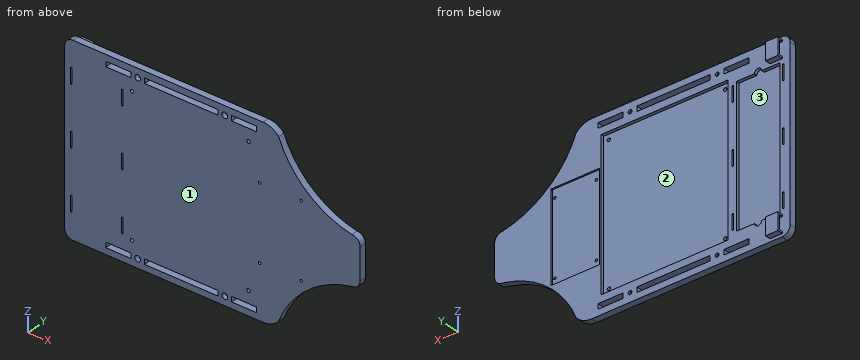
```python
from build123d import *

# Parameters (mm, degrees)
SALIENTE_EXTRUIR1_DEPTH = 6.35
CROQUIS2_R              = 1.825
CROQUIS2_W              = 63.849825594
CROQUIS2_H              = 5
CROQUIS2_W_2            = 24.299825594
CORTAR_EXTRUIR1_DEPTH   = 220.409920137
CORTAR_EXTRUIR2_DEPTH   = 3.175
CROQUIS4_W              = 45
CROQUIS4_H              = 80.85
CORTAR_EXTRUIR3_DEPTH   = 1.5
CROQUIS5_R              = 1.25
CORTAR_EXTRUIR4_DEPTH   = 220.371632292
CROQUIS7_W              = 44.995929737
CROQUIS7_H              = 3.9
CORTAR_EXTRUIR5_DEPTH   = 1.5
CROQUIS8_W              = 1.5
CROQUIS8_H              = 15
CORTAR_EXTRUIR6_DEPTH   = 220.409920137
CROQUIS9_W              = 123
CROQUIS9_H              = 144
CORTAR_EXTRUIR7_DEPTH   = 3.175
CROQUIS10_R             = 2.8
CORTAR_EXTRUIR8_DEPTH   = 4.35
CROQUIS11_R             = 1.65
CORTAR_EXTRUIR9_DEPTH   = 220.34099293
CROQUIS13_W             = 12.1
CROQUIS13_H             = 17
SALIENTE_EXTRUIR2_DEPTH = 5.5
CROQUIS14_W             = 13.5
CROQUIS14_H             = 3.5
CORTAR_EXTRUIR10_DEPTH  = 12.1
CROQUIS15_W             = 13.5
CROQUIS15_H             = 3.5
CORTAR_EXTRUIR11_DEPTH  = 12.1
CORTAR_EXTRUIR12_DEPTH  = 220.409920137
CORTAR_EXTRUIR15_DEPTH  = 1.5
CROQUIS19_W             = 7.395174406
CROQUIS19_H             = 5
CORTAR_EXTRUIR16_DEPTH  = 220.409920137


with BuildPart() as part:
    # Croquis1 → Saliente-Extruir1 (new body)
    with BuildSketch(Plane(origin=(0, 0, 0), x_dir=(1, 0, 0), z_dir=(0, 1, 0))):
        with BuildLine():
            Line((0, 0), (200, 0))
            Line((200, 0), (200, 15.2))
            ThreePointArc((200, 15.2), (197.701163079, 20.938172036), (191.9990235, 23.3249845))
            ThreePointArc((191.9990235, 23.3249845), (148.666739026, 44.032184001), (120.7781513, 83.1307986))
            ThreePointArc((120.7781513, 83.1307986), (113.982057966, 88.196272982), (105.7, 90))
            Line((105.7, 90), (0, 90))
            Line((0, 90), (-79, 90))
            ThreePointArc((-79, 90), (-84.638146896, 87.675499941), (-86.999825594, 82.052824894))
            Line((-86.999825594, 82.052824894), (-86.999825594, 41.494023494))
            ThreePointArc((-86.999825594, 41.494023494), (-92.052704294, 29.329564667), (-102.353503833, 21.119864881))
            ThreePointArc((-102.353503833, 21.119864881), (-108.040391417, 18.79326931), (-110.4, 13.12))
            Line((-110.4, 13.12), (-110.4, 0))
            Line((-110.4, 0), (0, 0))
        make_face()
    extrude(amount=SALIENTE_EXTRUIR1_DEPTH)

    # Simetría2: part across plane


with BuildPart() as part_1:
    add(part.part)
    add(part.part.mirror(Plane(origin=(0, 6.35, 0), x_dir=(1, 0, 0), z_dir=(0, 0, -1))))

    # Croquis2 → Cortar-Extruir1 (cut, through all)
    with BuildSketch(Plane(origin=(0, 6.35, 0), x_dir=(1, 0, 0), z_dir=(0, 1, 0))):
        with Locations(Location((68.5, 81.35, 0), (0, 0, 270))):
            Circle(CROQUIS2_R)
        with Locations(Location((-16.05, 81.35, 0), (0, 0, 270))):
            Circle(CROQUIS2_R)
        with Locations(Location((68.5, -81.35, 0), (0, 0, 90))):
            Circle(CROQUIS2_R)
        with Locations(Location((-16.05, -81.35, 0), (0, 0, 90))):
            Circle(CROQUIS2_R)
        with Locations((29.925087203, -81.35)):
            Rectangle(CROQUIS2_W, CROQUIS2_H)
        with Locations((-34.849912797, -81.35)):
            Rectangle(CROQUIS2_W_2, CROQUIS2_H)
        with Locations((87.299912797, -81.35)):
            Rectangle(CROQUIS2_W_2, CROQUIS2_H)
        with Locations((-34.849912797, 81.35)):
            Rectangle(CROQUIS2_W_2, CROQUIS2_H)
        with Locations((29.925087203, 81.35)):
            Rectangle(CROQUIS2_W, CROQUIS2_H)
        with Locations((87.299912797, 81.35)):
            Rectangle(CROQUIS2_W_2, CROQUIS2_H)
    extrude(amount=-CORTAR_EXTRUIR1_DEPTH, mode=Mode.SUBTRACT)

    # Croquis3 → Cortar-Extruir2 (cut)
    with BuildSketch(Plane(origin=(0, 6.35, 0), x_dir=(1, 0, 0), z_dir=(0, 1, 0))):
        with BuildLine():
            Line((-76.999825594, 67.375), (-59.324825594, 67.375))
            ThreePointArc((-59.324825594, 67.375), (-55.824825594, 70.875), (-52.324825594, 67.375))
            Line((-52.324825594, 67.375), (-34.649825594, 67.375))
            Line((-34.649825594, 67.375), (-34.649825594, -67.375))
            Line((-34.649825594, -67.375), (-52.324825594, -67.375))
            ThreePointArc((-52.324825594, -67.375), (-55.824825594, -70.875), (-59.324825594, -67.375))
            Line((-59.324825594, -67.375), (-76.999825594, -67.375))
            Line((-76.999825594, -67.375), (-76.999825594, 67.375))
        make_face()
    extrude(amount=-CORTAR_EXTRUIR2_DEPTH, mode=Mode.SUBTRACT)

    # Croquis4 → Cortar-Extruir3 (cut)
    with BuildSketch(Plane(origin=(0, 6.35, 0), x_dir=(1, 0, 0), z_dir=(0, 1, 0))):
        with Locations((122.5, 0)):
            Rectangle(CROQUIS4_W, CROQUIS4_H)
    extrude(amount=-CORTAR_EXTRUIR3_DEPTH, mode=Mode.SUBTRACT)

    # Croquis5 → Cortar-Extruir4 (cut, through all)
    with BuildSketch(Plane(origin=(0, 4.85, 0), x_dir=(1, 0, 0), z_dir=(0, 1, 0))):
        with Locations(Location((142.65, -34.175, 0), (0, 0, 270))):
            Circle(CROQUIS5_R)
        with Locations(Location((102.35, -34.175, 0), (0, 0, 90))):
            Circle(CROQUIS5_R)
        with Locations(Location((142.65, 38.075, 0), (0, 0, 270))):
            Circle(CROQUIS5_R)
        with Locations(Location((102.35, 38.075, 0), (0, 0, 90))):
            Circle(CROQUIS5_R)
    extrude(amount=-CORTAR_EXTRUIR4_DEPTH, mode=Mode.SUBTRACT)

    # Croquis7 → Cortar-Extruir5 (cut)
    with BuildSketch(Plane(origin=(0, 6.35, 0), x_dir=(1, 0, 0), z_dir=(0, 1, 0))):
        with Locations((122.497964869, 42.375)):
            Rectangle(CROQUIS7_W, CROQUIS7_H)
    extrude(amount=-CORTAR_EXTRUIR5_DEPTH, mode=Mode.SUBTRACT)

    # Croquis8 → Cortar-Extruir6 (cut, through all)
    with BuildSketch(Plane(origin=(0, 6.35, 0), x_dir=(1, 0, 0), z_dir=(0, 1, 0))):
        with Locations((-80.499825594, -57.5)):
            Rectangle(CROQUIS8_W, CROQUIS8_H)
        with Locations((-80.499825594, 57.5)):
            Rectangle(CROQUIS8_W, CROQUIS8_H)
        with Locations((-31.149825594, -57.5)):
            Rectangle(CROQUIS8_W, CROQUIS8_H)
        with Locations((-80.499825594, 0)):
            Rectangle(CROQUIS8_W, CROQUIS8_H)
        with Locations((-31.149825594, 0)):
            Rectangle(CROQUIS8_W, CROQUIS8_H)
        with Locations((-31.149825594, 57.5)):
            Rectangle(CROQUIS8_W, CROQUIS8_H)
    extrude(amount=-CORTAR_EXTRUIR6_DEPTH, mode=Mode.SUBTRACT)

    # Croquis9 → Cortar-Extruir7 (cut)
    with BuildSketch(Plane(origin=(0, 6.35, 0), x_dir=(1, 0, 0), z_dir=(0, 1, 0))):
        with Locations((35.100174406, 0)):
            Rectangle(CROQUIS9_W, CROQUIS9_H)
    extrude(amount=-CORTAR_EXTRUIR7_DEPTH, mode=Mode.SUBTRACT)

    # Croquis10 → Cortar-Extruir8 (cut)
    with BuildSketch(Plane.XZ):
        with Locations(Location((-16.05, 81.35, 0), (0, 0, 270))):
            Circle(CROQUIS10_R)
        with Locations(Location((-16.05, -81.35, 0), (0, 0, 90))):
            Circle(CROQUIS10_R)
        with Locations(Location((68.5, -81.35, 0), (0, 0, 270))):
            Circle(CROQUIS10_R)
        with Locations(Location((68.5, 81.35, 0), (0, 0, 90))):
            Circle(CROQUIS10_R)
    extrude(amount=-CORTAR_EXTRUIR8_DEPTH, mode=Mode.SUBTRACT)

    # Croquis11 → Cortar-Extruir9 (cut, through all)
    with BuildSketch(Plane(origin=(0, 3.175, 0), x_dir=(1, 0, 0), z_dir=(0, 1, 0))):
        with Locations(Location((-21.399825594, 67, 0), (0, 0, 270))):
            Circle(CROQUIS11_R)
        with Locations(Location((91.600174406, 67, 0), (0, 0, 90))):
            Circle(CROQUIS11_R)
        with Locations(Location((91.600174406, -67, 0), (0, 0, 270))):
            Circle(CROQUIS11_R)
        with Locations(Location((-21.399825594, -67, 0), (0, 0, 90))):
            Circle(CROQUIS11_R)
    extrude(amount=-CORTAR_EXTRUIR9_DEPTH, mode=Mode.SUBTRACT)

    # Croquis13 → Saliente-Extruir2 (add)
    with BuildSketch(Plane(origin=(0, 6.35, 0), x_dir=(1, 0, 0), z_dir=(0, 1, 0))):
        with Locations((-73.449825594, 78.6875)):
            Rectangle(CROQUIS13_W, CROQUIS13_H)
        with Locations((-73.449825594, -78.6875)):
            Rectangle(CROQUIS13_W, CROQUIS13_H)
    extrude(amount=SALIENTE_EXTRUIR2_DEPTH)

    # Croquis14 → Cortar-Extruir10 (cut)
    with BuildSketch(Plane.ZY.offset(79.499825594)):
        with Locations((78.6875, 8.1)):
            Rectangle(CROQUIS14_W, CROQUIS14_H)
    extrude(amount=-CORTAR_EXTRUIR10_DEPTH, mode=Mode.SUBTRACT)

    # Croquis15 → Cortar-Extruir11 (cut)
    with BuildSketch(Plane.ZY.offset(79.499825594)):
        with Locations((-78.6875, 8.1)):
            Rectangle(CROQUIS15_W, CROQUIS15_H)
    extrude(amount=-CORTAR_EXTRUIR11_DEPTH, mode=Mode.SUBTRACT)

    # Croquis16 → Cortar-Extruir12 (cut, through all)
    with BuildSketch(Plane(origin=(0, 6.35, 0), x_dir=(1, 0, 0), z_dir=(0, 1, 0))):
        Polygon((-86.999825594, 41.494023494), (-110.4, 41.494023494), (-110.4, 13.12), (-110.4, -13.12), (-110.4, -41.494023494), (-86.999825594, -41.494023494), align=None)
    extrude(amount=-CORTAR_EXTRUIR12_DEPTH, mode=Mode.SUBTRACT)

    # Croquis18 → Cortar-Extruir15 (cut)
    with BuildSketch(Plane(origin=(0, 6.35, 0), x_dir=(1, 0, 0), z_dir=(0, 1, 0))):
        Polygon((100, 44.325), (98, 44.325), (98, -42.425), (144.995929737, -42.425), (145, -40.425), (100, -40.425), align=None)
    extrude(amount=-CORTAR_EXTRUIR15_DEPTH, mode=Mode.SUBTRACT)

    # Croquis19 → Cortar-Extruir16 (cut, through all)
    with BuildSketch(Plane(origin=(0, 6.35, 0), x_dir=(1, 0, 0), z_dir=(0, 1, 0))):
        with Locations((-5.697412797, 81.35)):
            Rectangle(CROQUIS19_W, CROQUIS19_H)
        with Locations((-5.697412797, -81.35)):
            Rectangle(CROQUIS19_W, CROQUIS19_H)
    extrude(amount=-CORTAR_EXTRUIR16_DEPTH, mode=Mode.SUBTRACT)


solid = part_1.part
```
Work out the finished part from the listing and answer in its coordinate system (mm). Face numbers are marked on the shaded views. Give positions to 0.01 mm unless a question says otherwise; leave off trailing zeros. Loops run counter-clockwise (first coordinate to the right, second up) from the corner with the lowest first, then second, coordinate; pieces in that order, holes last. Notation, with made-up numbers: (3.25, 89.5) -> (36.25, 89.5) arc R23 ccw to (36.25, 117.5) -> close; hole circle Ø2 at (77.5, -39). An arc over 180 degrees is marked (long way). Put each result on its own line as item: value. Start each with the question number.
Item 1: The part is cut by section C-C (z = -33.5). Give the vertices of the cut face in (x, y) (3 decimals), then the cut area to 3 significant figures.
Item 2: Each of these flat-tipped pins is pushed along its axis until it touches: P1, Ø10, axis at x = -47, z = -40.5, coming from the +Y side (3 decimals); P2, Ø6, axis at x = 135.5, z = -60.5, coming from the +Y side; P3, Ø1.6, axis at x = -72.5, y = 10.5, coming from the -Z side; P4, Ø6, axis at x = -73, z = 79, coming from the -Y side. Where does it stop, or does it pass through?
Item 3: The part is cut by section A-A (x = 40.5). Give the vertices of the cut face in (y, z) (3 decimals).
Item 4: Find the intervals of material crossed by L1, parallel to X at y = 6, z = 0; L2, parallel to X at y = 3, z = -3; L3, parallel to Z at x = -70, y = 4 (3 decimals), in increasing order. Write a range as [from, to].
Item 5: The mould has two halves that part along Z. Classify the marked faces 1, 2 and 3: released by +Z, released by -Z, zero draft, split by the parting line, or undercut.
Item 6: The part is cut by section B-B (z = 75). Give the vertices of the cut face in (x, y).
Item 7: The part is cut by section D-D (z = 18.5). Give the vertices of the cut face in (x, y) (3 decimals), then the cut area to 3 significant figures.
Answers below:
1. outline: (-87, 0) -> (164.014, 0) -> (164.014, 6.35) -> (145, 6.35) -> (145, 4.85) -> (98, 4.85) -> (98, 6.35) -> (96.6, 6.35) -> (96.6, 3.175) -> (-26.4, 3.175) -> (-26.4, 6.35) -> (-34.65, 6.35) -> (-34.65, 3.175) -> (-77, 3.175) -> (-77, 6.35) -> (-87, 6.35) -> close
1. area: 998 mm2
2. P1: y = 3.175
2. P2: y = 6.35
2. P3: z = -87.19
2. P4: y = 0
3. outline: (0, -90) -> (6.35, -90) -> (6.35, -83.85) -> (0, -83.85) -> close; (0, -78.85) -> (6.35, -78.85) -> (6.35, -72) -> (3.175, -72) -> (3.175, 72) -> (6.35, 72) -> (6.35, 78.85) -> (0, 78.85) -> close; (0, 83.85) -> (6.35, 83.85) -> (6.35, 90) -> (0, 90) -> close
4. L1: [-87, -81.25], [-79.75, -77], [-34.65, -31.9], [-30.4, -26.4], [96.6, 98], [145, 200]
4. L2: [-87, -81.25], [-79.75, -31.9], [-30.4, 200]
4. L3: [-90, -67.375], [67.375, 90]
5. face 1: zero draft
5. face 2: undercut
5. face 3: undercut
6. outline: (-87, 0) -> (124.34, 0) -> (124.34, 6.35) -> (-87, 6.35) -> close; (-79.5, 9.85) -> (-67.4, 9.85) -> (-67.4, 11.85) -> (-79.5, 11.85) -> close
7. outline: (-87, 0) -> (199.344, 0) -> (199.344, 6.35) -> (145, 6.35) -> (145, 4.85) -> (98, 4.85) -> (98, 6.35) -> (96.6, 6.35) -> (96.6, 3.175) -> (-26.4, 3.175) -> (-26.4, 6.35) -> (-34.65, 6.35) -> (-34.65, 3.175) -> (-77, 3.175) -> (-77, 6.35) -> (-87, 6.35) -> close
7. area: 1,220 mm2
